Can you work these out from the drawing? Everything is in mm from the part's minimum corner. Give positions to 0.01 mm unless a question says otherwise; leave off trailing zeros. Loops run counter-clockwise (first coordinate to the right, second up) from the corner with the lowest first, then second, coordinate; pieces in that order, holes last.
Q1. I need wall thicknesses on line 1 (Z direction, x = 26, y = 1.55); line 2 (Z direction, x = 39.5, y = 0.95); line 3 (Z direction, x = 27, y = 0.75). Which ranges of each line are inside material? Lowest first, please.
Q2. If we section it at A-A (z = 15): Give the number of separate pieces and of enclosed holes in the cut face, plus the area to 3 significant figures.
Q3. If we section it at D-D (x = 24.5): Please give me the cut outline in (y, z), plus the area to 3 significant figures.
Q4. Will this pin go through, and if not, where does the flat tip stop? P1, Ø3.5, axis at x = 12.5, z = 15, coming from the +Y side.
Q5. If we section it at B-B (x = 12.5): Please give me the cut outline in (y, z).
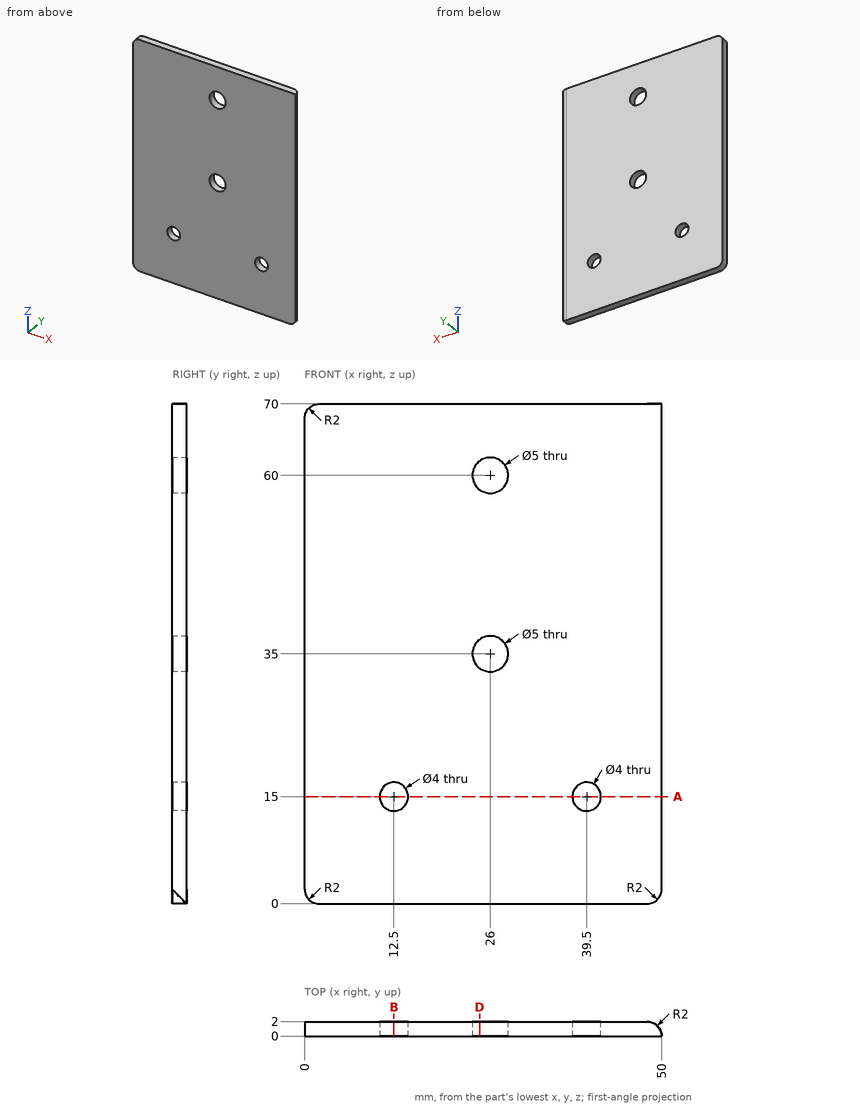
Check sheet entries:
1. line 1: z = 0 to 32.5, 37.5 to 57.5, 62.5 to 70
1. line 2: z = 0 to 13, 17 to 70
1. line 3: z = 0 to 32.71, 37.29 to 57.71, 62.29 to 70
2. separate pieces: 3
2. enclosed holes: 0
2. area: 83.1 mm2
3. outline: (0, 0) - (2, 0) - (2, 33) - (0, 33) - close; (0, 37) - (2, 37) - (2, 58) - (0, 58) - close; (0, 62) - (2, 62) - (2, 70) - (0, 70) - close
3. area: 124 mm2
4. P1: passes through
5. outline: (0, 0) - (2, 0) - (2, 13) - (0, 13) - close; (0, 17) - (2, 17) - (2, 70) - (0, 70) - close
